Geometry check sheet. Reference: the model listing, model coordinates, mm. Round coordinates to 2 decimals unless told otherwise and drop trailing zeros. Write each loop counter-clockwise with the first axis right and the second up, starting at its lowest first coordinate (ties: lowest second). Pieces come first, ordered by that corner, then holes.
Item 1: Cross-section at C-C (z = -5.5). Enter the section's corners in (x, y), then the cut area to 3 significant figures.
Item 2: Cross-section at B-B (y = -6). Enter the section's corners in (x, z), then the cut area to 3 significant figures.
Item 3: Depth check by flat-ended pin: P1, Ø4, axis at x = -65.5, y = 10, coming from the +Z side; P2, Ø5, axis at x = -96.5, y = 49.5, coming from the +Z side. Enter the tip coordinate at first touch or a pass-through.
Item 4: Scan lines: probe 1 along Z at (x, y) = (237.5, -20); probe 2 along Z at (x, y) = (-144, 21.5). Record each from-to range of solid material in increasing order.
Item 5: Cross-section at A-A (x = -106). Enter the section's corners in (y, z).
from build123d import *

# Parameters (mm, degrees)
F1_DEPTH = 582.041
F2_R     = 9.525
F3_R     = 9.525


with BuildPart() as f1:
    # F0 (on Right) → F1 (new body, symmetric)
    with BuildSketch(Plane.YZ):
        Polygon((4.234042, 0), (-33.865958, 0), (-33.865958, -1.27), (4.010107, -1.27), (37.964798, -13.628497), (63.470158, -22.911689), (63.904524, -21.718279), (40.036331, -13.030967), align=None)
    extrude(amount=F1_DEPTH, both=True)

    # F2
    f2_edges = [f1.edges().sort_by_distance(p)[0] for p in [
        (582.041, 63.687341, -22.314984),
    ]]
    fillet(f2_edges, radius=F2_R)

    # F3
    f3_edges = [f1.edges().sort_by_distance(p)[0] for p in [
        (-582.041, 63.687341, -22.314984),
    ]]
    fillet(f3_edges, radius=F3_R)


solid = f1.part
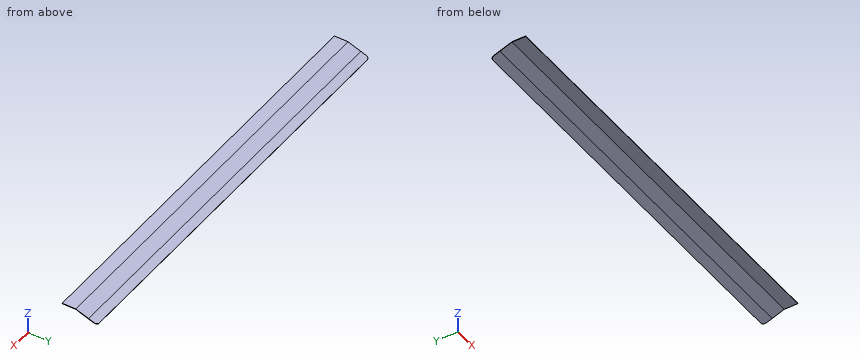
Resolved:
1. outline: (-582.04, 15.63) - (582.04, 15.63) - (582.04, 19.35) - (-582.04, 19.35) - close
1. area: 4,320 mm2
2. outline: (-582.04, -1.27) - (582.04, -1.27) - (582.04, 0) - (-582.04, 0) - close
2. area: 1,480 mm2
3. P1: stops at z = -1.37
3. P2: stops at z = -15.57
4. probe 1: z = -1.27 to 0
4. probe 2: z = -7.64 to -6.28
5. outline: (-33.87, -1.27) - (4.01, -1.27) - (63.47, -22.91) - (63.9, -21.72) - (4.23, 0) - (-33.87, 0) - close
